Build history of the part. All positions in model axes, mm. A direction names the side the tool comes from. Round coordinates to 2 decimals unless told otherwise and drop trailing zeros. Write each loop counter-clockwise with the first axis right and the second up, starting at its lowest first coordinate (ties: lowest second). Pieces come first, ordered by that corner, then holes. Notation, with made-up numbers: (36, 20) - (77, 20) arc R15 ccw to (77, 29) - close; hole circle Ø1 at (26.25, 71). An arc over 180 degrees is marked (long way). Answer as a JSON object with one key per item and string values. Group by question number.
Item 1: Which spindle directions (+Z, -Z, +X, -X, +Y, -Y) get a long thin tool onto all of the face, cutting with end or side? Do faces 5 (the flat face through (2, 13, 749.3)), 6 (the flat face through (15, 2.54, 369)). Say none if no direction does.
Item 2: Slice it at A-A, the plane x = 18.25. List the corners of the cut face in (y, z).
Item 3: Probe line 1 (Y direction, x = 22, z = 658); line 2 (X direction, y = 24.55, z = 165.1). List the from-to ranges inside material, lowest first. Write a range as from..to.
Item 4: Two-plate mould, pull along Y, no slides. Class faces 1 (the flat face through (15, 0, 369)), 2 (the flat face through (10, 25.4, 369)), 3 (the flat face through (0, 13, 369)), 4 (the cylindrical face through (24.112, 12.421, 730.244)): +Y half, -Y half, draft (parallel to the pull), parting line (faces both ways), or undercut.
Item 5: Slice it at B-B, the plane z = 73. List the corners of the cut face in (x, y).
Autodesk Inventor part; units mm, degrees
ref_plane "YZ Plane" through (0, 0, 0) normal (1, 0, 0) x (0, 1, 0)
ref_plane "XZ Plane" through (0, 0, 0) normal (0, 1, 0) x (-1, 0, 0)
ref_plane "XY Plane" through (0, 0, 0) normal (0, 0, 1) x (1, 0, 0)
sketch "Sketch1" plane through (0, 0, 0) normal (0, 0, 1) x (1, 0, 0)
  line L0 (0, 0) -> (25.4, 0)
  line L1 (25.4, 0) -> (25.4, 25.4)
  line L2 (25.4, 25.4) -> (0, 25.4)
  line L3 (0, 25.4) -> (0, 0)
  dimension "d0" = 25.4
  dimension "d1" = 25.4
extrude "Extrusion1" add sketch "Sketch1" along normal blind 749.3
shell "Shell1" thickness 2.54 removed faces 2 at (8.4667, 16.9333, 0) at (8.4667, 16.9333, 749.3)
sketch "Sketch2" plane through (0, 25.4, 0) normal (0, 1, 0) x (1, 0, 0)
  line L0 (25.4, 0) -> (0, 0)
  line L1 (0, 0) -> (0, -749.3)
  point P0 (12.7, -12.7)
  point P1 (12.7, -38.1)
  point P2 (12.7, -63.5)
  point P3 (12.7, -88.9)
  point P4 (12.7, -114.3)
  point P5 (12.7, -139.7)
  point P6 (12.7, -165.1)
  point P7 (12.7, -190.5)
  point P8 (12.7, -215.9)
  point P9 (12.7, -241.3)
  point P10 (12.7, -266.7)
  point P11 (12.7, -292.1)
  point P12 (12.7, -317.5)
  point P13 (12.7, -342.9)
  point P14 (12.7, -368.3)
  point P15 (12.7, -393.7)
  point P16 (12.7, -419.1)
  point P17 (12.7, -444.5)
  point P18 (12.7, -469.9)
  point P19 (12.7, -495.3)
  point P20 (12.7, -520.7)
  point P21 (12.7, -546.1)
  point P22 (12.7, -571.5)
  point P23 (12.7, -596.9)
  point P24 (12.7, -622.3)
  point P25 (12.7, -647.7)
  point P26 (12.7, -673.1)
  point P27 (12.7, -698.5)
  point P28 (12.7, -723.9)
  point P29 (12.7, -749.3)
  point P30 (12.7, -774.7)
  point P31 (12.7, -800.1)
  point P32 (12.7, -825.5)
  point P33 (12.7, -850.9)
  point P34 (12.7, -876.3)
  point P35 (12.7, -901.7)
  point P36 (12.7, -927.1)
  dimension "d5" = 12.7
  dimension "d6" = 12.7
  dimension "d9" = 25.4
hole "Hole1" at (12.7, 25.4, 12.7) at (12.7, 25.4, 38.1) at (12.7, 25.4, 63.5) at (12.7, 25.4, 88.9) at (12.7, 25.4, 114.3) at (12.7, 25.4, 139.7) at (12.7, 25.4, 165.1) at (12.7, 25.4, 190.5) at (12.7, 25.4, 215.9) at (12.7, 25.4, 241.3) at (12.7, 25.4, 266.7) at (12.7, 25.4, 292.1) at (12.7, 25.4, 317.5) at (12.7, 25.4, 342.9) at (12.7, 25.4, 368.3) at (12.7, 25.4, 393.7) at (12.7, 25.4, 419.1) at (12.7, 25.4, 444.5) at (12.7, 25.4, 469.9) at (12.7, 25.4, 495.3) at (12.7, 25.4, 520.7) at (12.7, 25.4, 546.1) at (12.7, 25.4, 571.5) at (12.7, 25.4, 596.9) at (12.7, 25.4, 622.3) at (12.7, 25.4, 647.7) at (12.7, 25.4, 673.1) at (12.7, 25.4, 698.5) at (12.7, 25.4, 723.9) at (12.7, 25.4, 749.3) at (12.7, 25.4, 774.7) at (12.7, 25.4, 800.1) at (12.7, 25.4, 825.5) at (12.7, 25.4, 850.9) at (12.7, 25.4, 876.3) at (12.7, 25.4, 901.7) direction (0, -1, 0) diameter 2.54 depth 50.8 tip angle 118
sketch "Sketch8" plane through (25.4, 0, 0) normal (1, 0, 0) x (0, 0, -1)
  line L0 (-749.3, 0) -> (-749.3, 25.4)
  line L1 (0, 25.4) -> (-749.3, 25.4)
  line L2 (0, 0) -> (0, 25.4)
  point P0 (-12.7, 12.7)
  point P1 (-723.9, 12.7)
  dimension "d57" = 25.4
  dimension "d58" = 12.7
  dimension "d59" = 12.7
  dimension "d60" = 12.7
hole "Hole5" at (25.4, 12.7, 12.7) at (25.4, 12.7, 723.9) direction (-1, 0, 0) diameter 12.7 depth 25.4 tip angle 118
properties part number "Support Pivs 25 upper" material "Aluminum 6061"
Geometry says:
{
 "1": {"face 5": "+Z, +X, -X, +Y, -Y", "face 6": "+Z, -Z"},
 "2": {"outline": "(0, 0) - (2.54, 0) - (2.54, 749.3) - (0, 749.3) - close; (22.86, 0) - (25.4, 0) - (25.4, 749.3) - (22.86, 749.3) - close"},
 "3": {"line 1": "y = 0..2.54, 22.86..25.4", "line 2": "x = 0..11.43, 13.97..25.4"},
 "4": {"face 1": "-Y half", "face 2": "+Y half", "face 3": "draft", "face 4": "undercut"},
 "5": {"outline": "(0, 0) - (25.4, 0) - (25.4, 25.4) - (0, 25.4) - close; hole (2.54, 2.54) - (22.86, 2.54) - (22.86, 22.86) - (2.54, 22.86) - close"}
}
